Part print with two shaded views. Sizes in mm from the minimum x, y, z corner. A direction names the side the tool comes from. Coordinates: 2 decimals unless noted, no trailing zeros. Loops run counter-clockwise (first coordinate to the right, second up) from the corner with the lowest first, then second, coordinate; pieces in that order, holes last. Notation, with made-up numbers: (12.5, -22.75) -> (67.5, -22.75) arc R7 cw to (67.5, -9.75) -> close; hole circle Ø7 at (44.25, 2.25). An arc over 180 degrees is marked (long way). Return JSON: item names as keys, results as strings. Group by question number.
(1) Saw through at A-A on z = 8.5. Write the cut outline in (x, y), then the cut area to 3 significant figures.
(2) Tool access for the marked faces 1 and 2: list every direction of +Z, -Z, +X, -X, +Y, -Y with a clear straight run to the whole face (end or side of a thin tool).
(3) Probe L1, parallel to Y at x = 10.75, z = 2.5; L2, parallel to Y at x = 4.5, z = 6.5 (1 decimal); L3, parallel to Z at x = 12.25, y = 6.25. List the from-to ranges inside material, lowest first.
(4) Saw through at D-D on y = 9.25. Write the cut outline in (x, z).
(5) Saw through at B-B on x = 1.5. Write the cut outline in (y, z) (1 decimal).
(6) Mould opens along Y. For the marked faces 3, 4 and 5 say: pulls with the +Y half, pulls with the -Y half, needs draft (parallel to the pull), parting line crosses it, or undercut.
(7) Flat gauge pins, fed straight in: pin 1 Ø6 at (y, z) = (22.5, 5.5) entering from -X; pin 2 Ø3 at (x, z) = (14, 3.5) entering from +Y; pin 3 Ø5.5 at (x, y) = (11.5, 11) entering from +Z; pin 4 Ø6 at (x, y) = (14, 16.5) entering from -Z. Where does each tip first touch, or does it go through?
(8) Saw through at C-C on x = 9. Write the cut outline in (y, z).
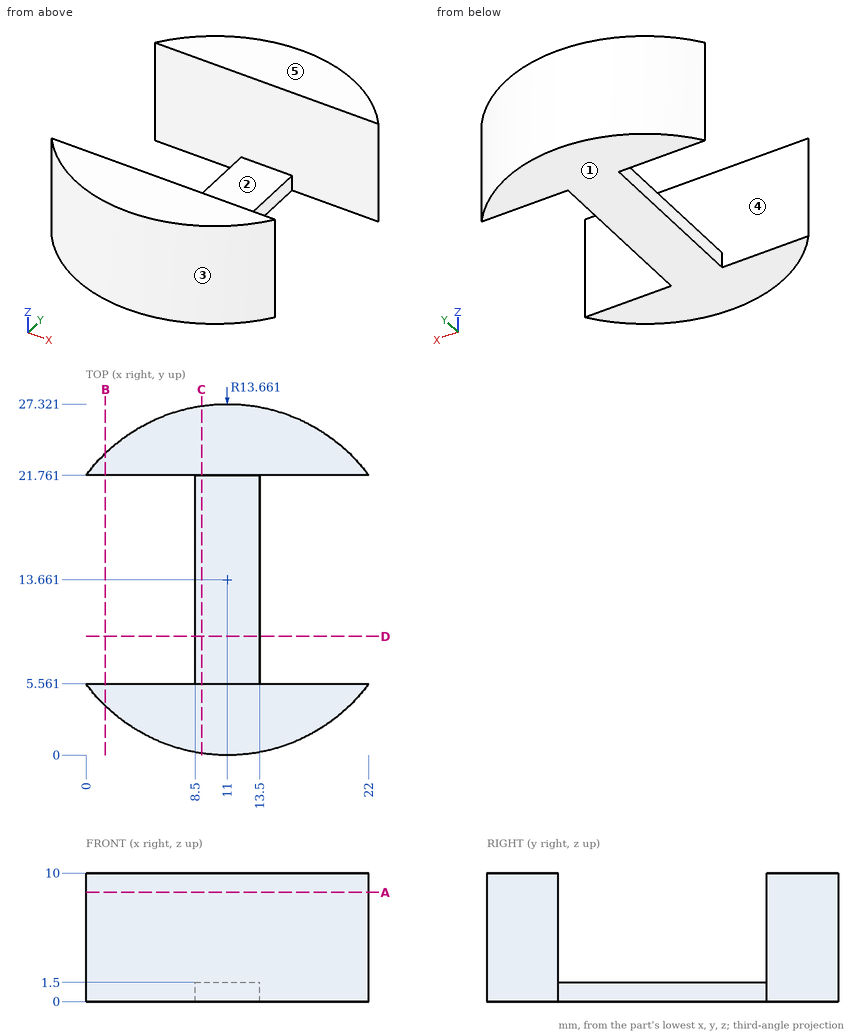
Geometry results:
{
 "1": {"outline": "(0, 5.56) arc R13.66 ccw to (22, 5.56) -> close; (0, 21.76) -> (22, 21.76) arc R13.66 ccw to start", "area": "171 mm²"},
 "2": {"face 1": "-Z, +X, -X, +Y, -Y", "face 2": "+Z, +X, -X"},
 "3": {"L1": "0 to 5.56, 21.76 to 27.32", "L2": "1.6 to 5.6, 21.8 to 25.7", "L3": "0 to 1.5"},
 "4": {"outline": "(8.5, 0) -> (13.5, 0) -> (13.5, 1.5) -> (8.5, 1.5) -> close"},
 "5": {"outline": "(3.8, 0) -> (5.6, 0) -> (5.6, 10) -> (3.8, 10) -> close; (21.8, 0) -> (23.5, 0) -> (23.5, 10) -> (21.8, 10) -> close"},
 "6": {"face 3": "pulls with the -Y half", "face 4": "undercut", "face 5": "needs draft"},
 "7": {"pin 1": "x = 0", "pin 2": "y = 27.24", "pin 3": "z = 1.5", "pin 4": "z = 0"},
 "8": {"outline": "(0.15, 0) -> (27.17, 0) -> (27.17, 10) -> (21.76, 10) -> (21.76, 1.5) -> (5.56, 1.5) -> (5.56, 10) -> (0.15, 10) -> close"}
}
